Read the model definition and answer for the solid it produces. Units are mm, in the model's axes. A direction names the side the tool comes from. Round coordinates to 2 decimals unless told otherwise and drop trailing zeros. Order: outer loops, then holes, each group sorted by start corner. A loop starts at its lowest first (then second) coordinate and runs counter-clockwise, first axis right, second up. Notation, with made-up numbers: (-10.5, 36) -> (21.5, 36) arc R32 ccw to (21.5, 64) -> close; hole circle Ø10 at (-17, -7.5). An arc over 180 degrees is marked (long way). Answer as a JSON object with one key per item and string values. Group by question number.
Item 1: Given P1, Ø20, axis at x = -7.5, y = -4.5, coming from the +Z side, flat-ended and moving along its own axis, determine where the tip first touches the part or whether it passes through.
Item 2: Section B-B, the plane y = -13.5 is taken. Write down the section's boundary in (x, z), plus the area to 3 significant figures.
Item 3: The mould has two halves that part along Y. Classify faces 4 (the flat face through (55.838, -6, -2)), 5 (the flat face through (5, -35.228, -2)), 6 (the flat face through (-19, -5, -3)): pulls with the +Y half, pulls with the -Y half, needs draft (parallel to the pull), parting line crosses it, or undercut.
Item 4: For faces 1 (the flat face through (0, -14.581, -3)), 2 (the flat face through (5, 24.772, -2)), 3 (the flat face through (3, -17, -1)), determine the directions among +Z, -Z, +X, -X, +Y, -Y from which every point of the face is accessible in a straight line to the end or side of a thin tool.
Item 5: Section C-C, the plane z = -2.65 is taken. Write down the section's boundary in (x, y).
Item 6: Section A-A, the plane x = 18 is taken. Write down the section's boundary in (y, z).
Item 7: Consider probe 1 along Y at (x, z) = (-8.5, -0.55); probe 2 along Y at (x, z) = (-10.5, -1.8); probe 3 along X at (y, z) = (-11.5, -4.35). Determine where each line is inside the solid, lowest interval first. Write a range as from..to.
from build123d import *

# Parameters (mm, degrees)
F0_W     = 100
F0_H     = 60
F3_DEPTH = 5
F1_W     = 48
F1_H     = 25
F4_DEPTH = 1
F2_W     = 38
F2_H     = 20
F5_DEPTH = 10


with BuildPart() as f3:
    # F0 (on Top) → F3 (new body)
    with BuildSketch(Plane.XY):
        with Locations((5.838281, -5.227597)):
            Rectangle(F0_W, F0_H)
    extrude(amount=-F3_DEPTH)

    # F1 (on Top) → F4 (cut)
    with BuildSketch(Plane.XY):
        with Locations((1.309254, -6.3852)):
            Rectangle(F1_W, F1_H)
    extrude(amount=-F4_DEPTH, mode=Mode.SUBTRACT)

    # F2 (on face) → F5 (cut)
    with BuildSketch(Plane.XY):
        with Locations((0, -4.581108)):
            Rectangle(F2_W, F2_H)
    extrude(amount=-F5_DEPTH, mode=Mode.SUBTRACT)


solid = f3.part
Values found:
{
 "1": {"P1": "z = -1"},
 "2": {"outline": "(-44.16, -5) -> (-19, -5) -> (-19, -1) -> (-22.69, -1) -> (-22.69, 0) -> (-44.16, 0) -> close; (19, -5) -> (55.84, -5) -> (55.84, 0) -> (25.31, 0) -> (25.31, -1) -> (19, -1) -> close", "area": "300 mm2"},
 "3": {"face 4": "needs draft", "face 5": "pulls with the -Y half", "face 6": "undercut"},
 "4": {"face 1": "+Z, -Z", "face 2": "+Z, -Z, +X, -X, +Y", "face 3": "+Z"},
 "5": {"outline": "(-44.16, -35.23) -> (55.84, -35.23) -> (55.84, 24.77) -> (-44.16, 24.77) -> close; hole (-19, -14.58) -> (19, -14.58) -> (19, 5.42) -> (-19, 5.42) -> close"},
 "6": {"outline": "(-35.23, -5) -> (-14.58, -5) -> (-14.58, -1) -> (-18.89, -1) -> (-18.89, 0) -> (-35.23, 0) -> close; (5.42, -5) -> (24.77, -5) -> (24.77, 0) -> (6.11, 0) -> (6.11, -1) -> (5.42, -1) -> close"},
 "7": {"probe 1": "-35.23..-18.89, 6.11..24.77", "probe 2": "-35.23..-14.58, 5.42..24.77", "probe 3": "-44.16..-19, 19..55.84"}
}
